from build123d import *

# Parameters (mm, degrees)
IZIM1_W                     = 40
IZIM1_H                     = 20
Y_KSEKLIK_EKSTR_ZYON1_DEPTH = 5
IZIM2_R                     = 2.6
KES_EKSTR_ZYON1_DEPTH       = 5
PAH1_SIZE                   = 1


with BuildPart() as part:
    # Çizim1 → Yükseklik-Ekstrüzyon1 (new body)
    with BuildSketch(Plane.XY):
        with Locations((-51.29829922, 6.046511628)):
            Rectangle(IZIM1_W, IZIM1_H)
    extrude(amount=Y_KSEKLIK_EKSTR_ZYON1_DEPTH)

    # Çizim2 → Kes-Ekstrüzyon1 (cut)
    with BuildSketch(Plane.XY.offset(5)):
        with Locations((-61.29829922, 5.367137417)):
            Circle(IZIM2_R)
        with Locations((-41.29829922, 5.367137417)):
            Circle(IZIM2_R)
    extrude(amount=-KES_EKSTR_ZYON1_DEPTH, mode=Mode.SUBTRACT)

    # Pah1
    pah1_edges = [part.edges().sort_by_distance(p)[0] for p in [
        (-63.89829922, 5.367137417, 0),
        (-63.89829922, 5.367137417, 5),
        (-43.89829922, 5.367137417, 0),
        (-43.89829922, 5.367137417, 5),
    ]]
    chamfer(pah1_edges, length=PAH1_SIZE)


solid = part.part
The listing builds one solid part. Answer for the finished solid, in the listing's coordinates (mm). Give positions to 0.01 mm unless a question says otherwise; leave off trailing zeros. Write each loop counter-clockwise with the first axis right and the second up, starting at its lowest first coordinate (ties: lowest second). Pieces come first, ordered by that corner, then holes.
Item 1: Section A-A, the plane z = 1.5 is taken. Write down the section's boundary in (x, y), plus the area to 3 significant figures.
Item 2: Section B-B, the plane y = 7.25 is taken. Count the separate pieces of the cut face and the enclosed holes in it, plus the area to 3 significant figures.
Item 3: A flat-ended cylindrical pin translates along its axis: P1, Ø7, axis at x = -61.3, y = 5.37, coming from the -Z side. Find the tip coordinate at first contact, or state that the pin passes through.
Item 4: Find the intervals of material crossed by line 1 along X through (y, z) = (5.5, 0.85); line 2 along Y through (x, z) = (-61.5, 0.65); line 3 along X through (y, z) = (4.5, 1.75), in increasing order.
Item 5: Determine the mould class of faces 1 (the flat face through (-71.298, 6, 2)), 2 (the flat face through (-52, 16.047, 2)), 3 (the cylindrical face through (-63.362, 3.785, 2.521)) for opening direction X: released by +X, released by -X, zero draft, split by the parting line, or undercut.
Completed:
1. outline: (-71.3, -3.95) - (-31.3, -3.95) - (-31.3, 16.05) - (-71.3, 16.05) - close; hole circle Ø5.2 at (-61.3, 5.37); hole circle Ø5.2 at (-41.3, 5.37)
1. area: 758 mm2
2. separate pieces: 3
2. enclosed holes: 0
2. area: 159 mm2
3. P1: stops at z = 0.1
4. line 1: x = -71.3 to -64.05, -58.55 to -44.05, -38.55 to -31.3
4. line 2: y = -3.95 to 2.42, 8.31 to 16.05
4. line 3: x = -71.3 to -63.75, -58.85 to -43.75, -38.85 to -31.3
5. face 1: released by -X
5. face 2: zero draft
5. face 3: undercut
